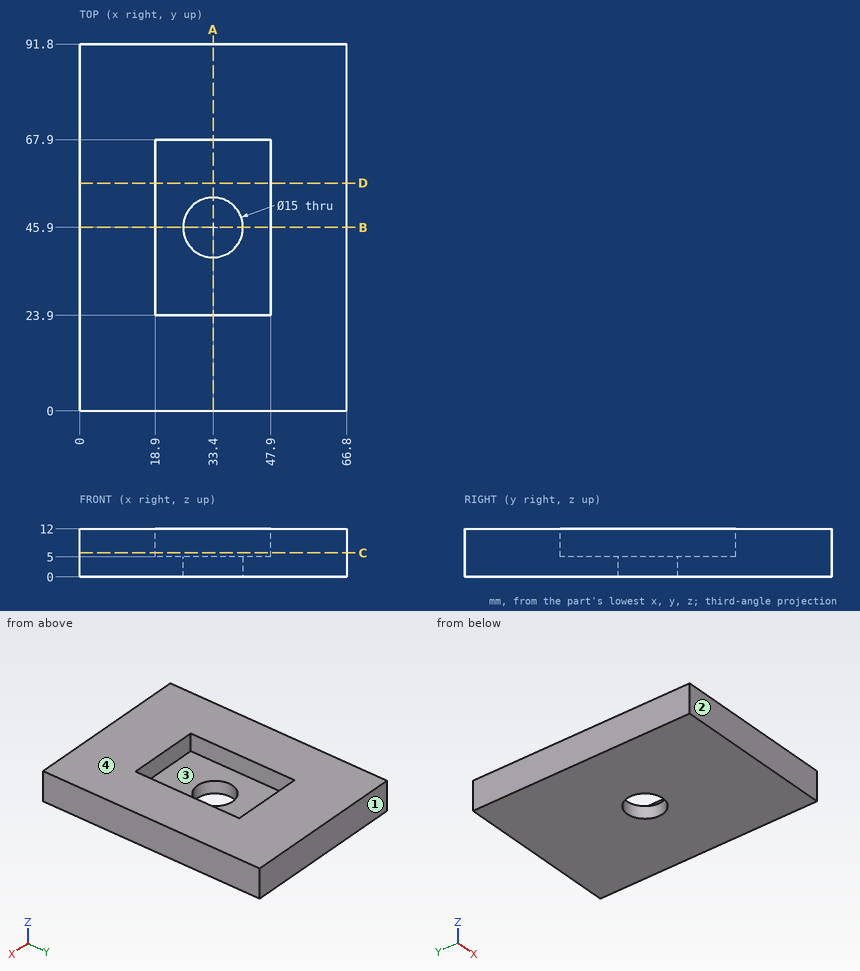
Answer from the drawing. Dimensions are ordinates in mm from the lowest x, y and z of the part. Coordinates: 2 decimals unless noted, no trailing zeros. Loops run counter-clockwise (first coordinate to the right, second up) from the corner with the lowest first, then second, coordinate; pieces in that order, holes last. Notation, with made-up numbers: (-9, 79) - (34, 79) arc R7 cw to (34, 88) - close; hole circle Ø1 at (63, 65.5). An arc over 180 degrees is marked (long way). Answer in a Markdown table with one row per item.
1. Find section D-D, the plane y = 57. Write down the section's boundary in (x, z).
Conclusion:
| item | result |
|---|---|
| outline | (0, 0) - (66.8, 0) - (66.8, 12) - (47.9, 12) - (47.9, 5) - (18.9, 5) - (18.9, 12) - (0, 12) - close |
2. Straight lines are drawn through the part: line 1 (X direction, y = 41, z = 10.5); line 2 (Y direction, x = 33.4, z = 3.35); line 3 (Y direction, x = 42, z = 10). For each, find the intervals that lie inside material, in ascending order.
Conclusion:
| item | result |
|---|---|
| line 1 | x = 0 to 18.9, 47.9 to 66.8 |
| line 2 | y = 0 to 38.4, 53.4 to 91.8 |
| line 3 | y = 0 to 23.9, 67.9 to 91.8 |
3. Determine the mould class of the marked faces 1, 2, 3 and 4 for opening direction Y: +Y half, -Y half, draft (parallel to the pull), parting line (faces both ways), or undercut.
Conclusion:
| item | result |
|---|---|
| face 1 | +Y half |
| face 2 | -Y half |
| face 3 | undercut |
| face 4 | draft |
4. Find section A-A, the plane x = 33.4. Write down the section's boundary in (y, z).
Conclusion:
| item | result |
|---|---|
| outline | (0, 0) - (38.4, 0) - (38.4, 5) - (23.9, 5) - (23.9, 12) - (0, 12) - close; (53.4, 0) - (91.8, 0) - (91.8, 12) - (67.9, 12) - (67.9, 5) - (53.4, 5) - close |
5. Find section C-C, the plane z = 6. Write down the section's boundary in (x, y).
Conclusion:
| item | result |
|---|---|
| outline | (0, 0) - (66.8, 0) - (66.8, 91.8) - (0, 91.8) - close; hole (18.9, 23.9) - (47.9, 23.9) - (47.9, 67.9) - (18.9, 67.9) - close |
6. Find section B-B, the plane y = 45.9. Write down the section's boundary in (x, z), then the cut area to 3 significant figures.
Conclusion:
| item | result |
|---|---|
| outline | (0, 0) - (25.9, 0) - (25.9, 5) - (18.9, 5) - (18.9, 12) - (0, 12) - close; (40.9, 0) - (66.8, 0) - (66.8, 12) - (47.9, 12) - (47.9, 5) - (40.9, 5) - close |
| area | 524 mm² |
